The drawing under review shows one solid part. Ordinate dimensions are in mm from its lowest x, y, z. A direction names the side the tool comes from. Coordinates: 2 decimals unless noted, no trailing zeros. Loops run counter-clockwise (first coordinate to the right, second up) from the corner with the lowest first, then second, coordinate; pieces in that order, holes last. Notation, with made-up numbers: M 81.5,37.25 L 137.5,37.25 A31 ccw 137.5,75.25 Z; hole C -30,70 d3. An arc over 180 degrees is marked long. Answer as a JSON object with one key per item and string values. Group by question number.
1. Consider section A-A (x = 19). State the section outline as (y, z) points.
2. To check wall thickness, follow probe 1 along Y at (x, z) = (16, 7.75); probe 2 along X at (y, z) = (22, 2); probe 3 along X at (y, z) = (17.5, 2). State the ranges of each line that lie inside material, in increasing order.
3. Consider section C-C (y = 10). State the section outline as (x, z) points.
4. Machinability: for the marked faces 1, 2, 3, 4 and 5, which of the approach directions +Z, -Z, +X, -X, +Y, -Y give a long, thin tool a straight path to every point of the face, cutting with its end or side? Answer none if there is none.
5. Consider section B-B (z = 2.75). Count the separate pieces of the cut face and the enclosed holes in it, then the cut area to 3 significant figures.
6. Insertion check: pin 1 (1.1 mm diameter, centred on x = 46, z = 5, fed in from -Y); pin 2 (2 mm diameter, centred on x = 20.5, z = 2.5, fed in from +Y); pin 3 (1.5 mm diameter, centred on y = 33, z = 5, fed in from -X); pin 4 (5 mm diameter, centred on x = 16.5, y = 22.5, fed in from -Z). Each pin has a flat end and moves straight along its axis. Give the tip position at first contact, or say it passes through.
7. Draft analysis for pull direction X (two halves, no side actions). For the marked faces 6, 7 and 8, state which applies: +X half, -X half, draft (parallel to the pull), parting line (faces both ways), or undercut.
8. Consider section D-D (y = 37). State the section outline as (x, z) points.
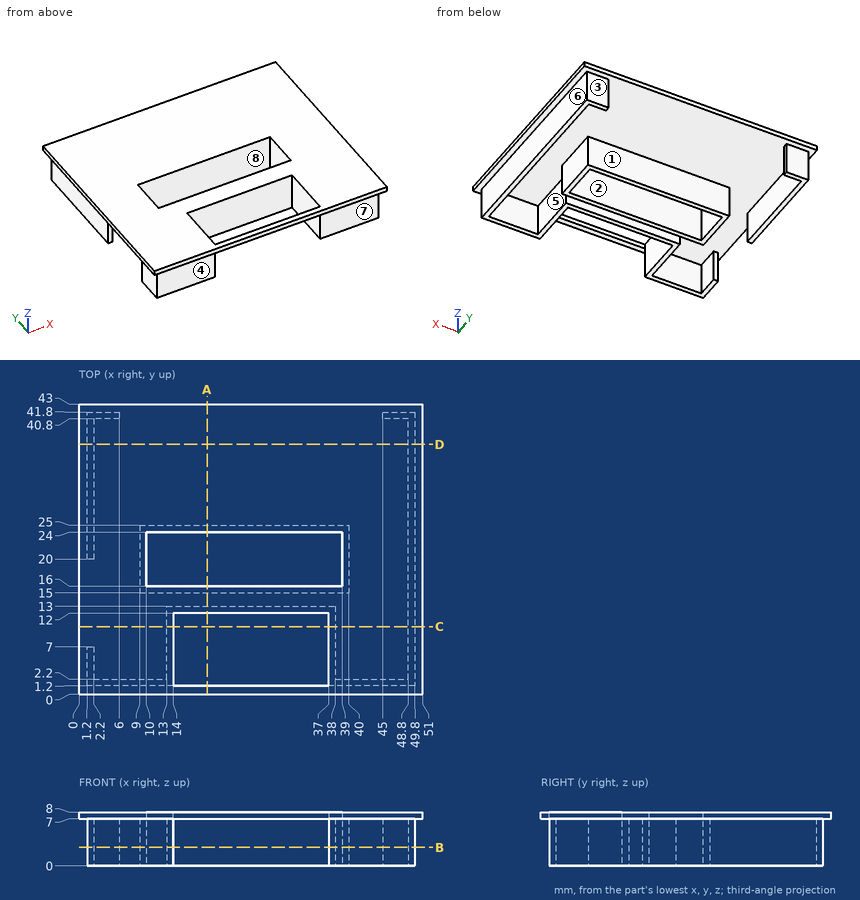
Findings below:
{
 "1": {"outline": "M 0,7 L 1.2,7 L 1.2,8 L 0,8 Z; M 12,0 L 13,0 L 13,7 L 15,7 L 15,0 L 16,0 L 16,8 L 12,8 Z; M 24,0 L 25,0 L 25,7 L 43,7 L 43,8 L 24,8 Z"},
 "2": {"probe 1": "y = 0 to 1.2, 12 to 16, 24 to 43", "probe 2": "x = 1.2 to 2.2, 9 to 10, 39 to 40, 48.8 to 49.8", "probe 3": "x = 9 to 10, 39 to 40, 48.8 to 49.8"},
 "3": {"outline": "M 0,7 L 13,7 L 13,0 L 14,0 L 14,8 L 0,8 Z; M 37,0 L 38,0 L 38,7 L 48.8,7 L 48.8,0 L 49.8,0 L 49.8,7 L 51,7 L 51,8 L 37,8 Z"},
 "4": {"face 1": "-Z, +Y", "face 2": "+Z, -Z", "face 3": "-Z, +X, -X, +Y", "face 4": "-Z, +X, -X, -Y", "face 5": "-Z"},
 "5": {"separate pieces": "3", "enclosed holes": "1", "area": "222 mm^2"},
 "6": {"pin 1": "stops at y = 1.2", "pin 2": "stops at y = 25", "pin 3": "stops at x = 1.2", "pin 4": "stops at z = 0"},
 "7": {"face 6": "+X half", "face 7": "draft", "face 8": "undercut"},
 "8": {"outline": "M 0,7 L 1.2,7 L 1.2,0 L 2.2,0 L 2.2,7 L 48.8,7 L 48.8,0 L 49.8,0 L 49.8,7 L 51,7 L 51,8 L 0,8 Z"}
}
